Could you check a few things on this model? Use its own coordinates, in mm. A direction names the side the tool comes from. Coordinates: 2 decimals unless noted, no trailing zeros. Order: outer loops, then holes, each group sorted by start corner. A loop starts at its lowest first (then second) coordinate and runs counter-clockwise, first axis right, second up. Notation, with made-up numbers: (62.5, 62) - (92.5, 62) arc R26 ccw to (92.5, 93) - close; hole circle Ø2 at (-33, -11.5). An arc over 180 degrees is marked (long way). One line per item, written item: value. Start each with the question number.
from build123d import *

# Parameters (mm, degrees)
BOX033_W           = 20
BOX033_H           = 20
BOX033_DEPTH       = 280
BOX034_W           = 20
BOX034_H           = 20
BOX034_DEPTH       = 280
BOX031_W           = 20
BOX031_H           = 20
BOX031_DEPTH       = 280
BOX032_W           = 20
BOX032_H           = 20
BOX032_DEPTH       = 280
BOX029_W           = 20
BOX029_H           = 20
BOX029_DEPTH       = 280
BOX030_W           = 20
BOX030_H           = 20
BOX030_DEPTH       = 280
BOX027_W           = 20
BOX027_H           = 20
BOX027_DEPTH       = 280
BOX028_W           = 20
BOX028_H           = 20
BOX028_DEPTH       = 280
BOX035_W           = 20
BOX035_H           = 20
BOX035_DEPTH       = 480
BOX035_PITCH_ANGLE = 90


with BuildPart() as box033:
    # Box033 → Box033 (new body)
    with BuildSketch(Plane(origin=(70, 10, 760), x_dir=(1, 0, 0), z_dir=(0, 0, 1))):
        with Locations((10, 10)):
            Rectangle(BOX033_W, BOX033_H)
    extrude(amount=BOX033_DEPTH)


with BuildPart() as box034:
    # Box034 → Box034 (new body)
    with BuildSketch(Plane(origin=(410, 10, 760), x_dir=(1, 0, 0), z_dir=(0, 0, 1))):
        with Locations((10, 10)):
            Rectangle(BOX034_W, BOX034_H)
    extrude(amount=BOX034_DEPTH)


with BuildPart() as box031:
    # Box031 → Box031 (new body)
    with BuildSketch(Plane(origin=(50, 10, 510), x_dir=(1, 0, 0), z_dir=(0, 0, 1))):
        with Locations((10, 10)):
            Rectangle(BOX031_W, BOX031_H)
    extrude(amount=BOX031_DEPTH)


with BuildPart() as box032:
    # Box032 → Box032 (new body)
    with BuildSketch(Plane(origin=(430, 10, 510), x_dir=(1, 0, 0), z_dir=(0, 0, 1))):
        with Locations((10, 10)):
            Rectangle(BOX032_W, BOX032_H)
    extrude(amount=BOX032_DEPTH)


with BuildPart() as box029:
    # Box029 → Box029 (new body)
    with BuildSketch(Plane(origin=(30, 10, 260), x_dir=(1, 0, 0), z_dir=(0, 0, 1))):
        with Locations((10, 10)):
            Rectangle(BOX029_W, BOX029_H)
    extrude(amount=BOX029_DEPTH)


with BuildPart() as box030:
    # Box030 → Box030 (new body)
    with BuildSketch(Plane(origin=(450, 10, 260), x_dir=(1, 0, 0), z_dir=(0, 0, 1))):
        with Locations((10, 10)):
            Rectangle(BOX030_W, BOX030_H)
    extrude(amount=BOX030_DEPTH)


with BuildPart() as box027:
    # Box027 → Box027 (new body)
    with BuildSketch(Plane(origin=(10, 10, 10), x_dir=(1, 0, 0), z_dir=(0, 0, 1))):
        with Locations((10, 10)):
            Rectangle(BOX027_W, BOX027_H)
    extrude(amount=BOX027_DEPTH)


with BuildPart() as box028:
    # Box028 → Box028 (new body)
    with BuildSketch(Plane(origin=(470, 10, 10), x_dir=(1, 0, 0), z_dir=(0, 0, 1))):
        with Locations((10, 10)):
            Rectangle(BOX028_W, BOX028_H)
    extrude(amount=BOX028_DEPTH)


with BuildPart() as solar_panel_supporter:
    # Box035 → Box035 (new body)
    with BuildSketch(Plane.XY):
        with Locations((10, 10)):
            Rectangle(BOX035_W, BOX035_H)
    extrude(amount=BOX035_DEPTH)


with BuildPart() as solar_panel_supporter_1:
    # Box035 pitch: moved
    add(solar_panel_supporter.part.rotate(Axis((0, 0, 0), (0, 1, 0)), BOX035_PITCH_ANGLE))


with BuildPart() as solar_panel_supporter_2:
    # Box035 placement: moved
    add(solar_panel_supporter_1.part.moved(Location((10, 10, 1060))))

    # Fusion013: union Box033, Box034, Box031, Box032, Box029, Box030, Box027, Box028
    add(box033.part)
    add(box034.part)
    add(box031.part)
    add(box032.part)
    add(box029.part)
    add(box030.part)
    add(box027.part)
    add(box028.part)


solid = solar_panel_supporter_2.part
Q1. If I drill on L1, parallel to X at y = 11.5, z = 547; L2, parallel to X at y = 23.75, z = 274; L3, parallel to Z at x = 444, y = 11.5, over which ranges is the centre line in solid material (lowest first)?
Q2. I'm going to push flat-ended pins straight in: pin 1 (1.5 mm diameter, centred on y = 27, z = 882, fed in from +X); pin 2 (1 mm diameter, centred on y = 21, z = 352.5, fed in from -X); pin 3 (10 mm diameter, centred on y = 15.5, z = 394, fed in from +X). Where does each tip first touch, or does it pass through?
Q3. I want a section at B-B on x = 302. Please give me the cut outline in (y, z), then the cut area to 3 significant figures.
Q4. Which directions (+Z, -Z, +X, -X, +Y, -Y) give clear straight access to the entire face, cutting with the end or side of a thin tool? Please do faces 4 (the flat face through (10, 20, 148)), 5 (the flat face through (60, 20, 510)), 6 (the flat face through (490, 20, 148)), 7 (the flat face through (40, 20, 540)), 8 (the flat face through (460, 20, 540)).
Q5. We'd pull the mould along Z, two halves only. Please class faces 1 (the flat face through (430, 20, 913)), 2 (the flat face through (470, 20, 133)), 3 (the flat face through (480, 20, 10)): +Z half, -Z half, draft (parallel to the pull), parting line (faces both ways), or undercut.
Q6. I want a section at A-A on z = 936. Please give me the cut outline in (x, y), then the cut area to 3 significant figures.
Values follow:
1. L1: x = 50 to 70, 430 to 450
1. L2: x = 10 to 50, 450 to 490
1. L3: z = 510 to 790, 1040 to 1060
2. pin 1: stops at x = 430
2. pin 2: stops at x = 30
2. pin 3: stops at x = 470
3. outline: (10, 1040) - (30, 1040) - (30, 1060) - (10, 1060) - close
3. area: 400 mm^2
4. face 4: +Z, -Z, -X, +Y, -Y
4. face 5: -Z, +Y, -Y
4. face 6: +Z, -Z, +X, +Y, -Y
4. face 7: -X, +Y, -Y
4. face 8: +X, +Y, -Y
5. face 1: undercut
5. face 2: draft
5. face 3: -Z half
6. outline: (70, 10) - (90, 10) - (90, 30) - (70, 30) - close; (410, 10) - (430, 10) - (430, 30) - (410, 30) - close
6. area: 800 mm^2
